from build123d import *

# Parameters (mm, degrees)
F4_R     = 0.621052
F5_DEPTH = 25.4


with BuildPart() as f3:
    # F0 (on Top) → F3 section 0
    with BuildSketch(Plane.XY):
        with BuildLine():
            ThreePointArc((0, 18.184091), (-4.48363, -0.639026), (-2.805989, -19.915909))
            Line((-2.805989, -19.915909), (2.85146, -19.915909))
            ThreePointArc((2.85146, -19.915909), (4.506652, -0.635328), (0, 18.184091))
        make_face()
    # F2 (on offset) → F3 section 1
    with BuildSketch(Plane.XY.offset(25.4)):
        with BuildLine():
            ThreePointArc((0, 34.804691), (-10.264244, 5.338028), (-7.867152, -25.77295))
            Line((-7.867152, -25.77295), (7.245407, -25.77295))
            ThreePointArc((7.245407, -25.77295), (9.944669, 5.272011), (0, 34.804691))
        make_face()
    loft()

    # F4 (on face) → F5 (join)
    with BuildSketch(Plane.XY.offset(25.4)):
        with Locations((0, 7.182024)):
            Circle(F4_R)
    extrude(amount=F5_DEPTH)

    # F9: sweep along a path in F8
    with BuildLine(Plane.YZ) as f9_path:
        ThreePointArc((6.253172, 36.976661), (10.944831, 43.26766), (8.742062, 50.8))
    # F7 (on offset) → F9 (sweep)
    with BuildSketch(Plane.XY.offset(50.8)):
        with BuildLine():
            ThreePointArc((-10.597052, 4.972847), (0, 7.3424), (10.597052, 4.972847))
            Line((10.597052, 4.972847), (10.597052, 6.139166))
            ThreePointArc((10.597052, 6.139166), (0, 8.742062), (-10.597052, 6.139166))
            Line((-10.597052, 6.139166), (-10.597052, 4.972847))
        make_face()
    sweep(path=f9_path.line)


solid = f3.part
Read the model definition and answer for the solid it produces. Units are mm, in the model's axes. A direction names the side the tool comes from. Coordinates: 2 decimals unless noted, no trailing zeros. Write each loop counter-clockwise with the first axis right and the second up, starting at its lowest first coordinate (ties: lowest second). Pieces come first, ordered by that corner, then holes. Notation, with made-up numbers: (1, 49.25) -> (41, 49.25) arc R16 ccw to (41, 67.25) -> close; hole circle Ø10 at (-36.75, 10). An arc over 180 degrees is marked (long way). Return JSON: item names as keys, results as strings.
(1) The part is cut by section A-A on z = 29. Give the vertices of the cut face in (x, y).
Answers below:
{"outline": "circle Ø1.24 at (0, 7.18)"}
(2) Consider line 1 along Z through (x, y) = (-0.5, -8.5); line 2 along Y through (x, z) = (6, 41.5); line 3 along X through (y, z) = (1, 9). Determine where each line is inside the solid, lowest interval first. Write a range as from..to.
Answers below:
{"line 1": "0..25.4", "line 2": "8.87..9.81", "line 3": "-6.58..6.48"}
(3) Each of these flat-tipped pins is pushed along its axis until it touches: P1, Ø8, axis at x = -3.5, z = 33, coming from the -Y side; P2, Ø1.5, axis at x = 2.5, y = -8.5, coming from the +Z side; P3, Ø8, axis at x = 7, y = -2.5, coming from the -Z side; P4, Ø2, axis at y = 7, z = 45, coming from the -X side. Where does it stop, or does it pass through?
Answers below:
{"P1": "y = 6.56", "P2": "z = 25.4", "P3": "z = 0", "P4": "x = -0.62"}
(4) For a pull along Z with two mould halves and no side action, classify faces 4 (the flat face through (1, -2, 0)), 5 (the cylindrical face through (-0.081, 7.798, 31.6)), 6 (the flat face through (-10.597, 9, 46)) as pulls with the +Z half, pulls with the -Z half, needs draft (parallel to the pull), parting line crosses it, or undercut.
Answers below:
{"face 4": "pulls with the -Z half", "face 5": "undercut", "face 6": "needs draft"}
(5) Which of the six approach directions +Z, -Z, +X, -X, +Y, -Y give full straight-line access (tool end or side, diameter ignored) to faces 1 (the flat face through (0.15, 6.42, 37.56)), 2 (the flat face through (10.597, 9, 45)), 3 (the cylindrical face through (-0.135, 6.576, 44.328))?
Answers below:
{"face 1": "-Y", "face 2": "+Z, -Z, +X, +Y, -Y", "face 3": "none"}
